Build history of the part. All positions in model axes, mm. A direction names the side the tool comes from. Give positions to 0.01 mm unless a question says otherwise; leave off trailing zeros. Loops run counter-clockwise (first coordinate to the right, second up) from the corner with the lowest first, then second, coordinate; pieces in that order, holes last. Notation, with made-up numbers: (-24.75, 88) -> (31.25, 88) arc R26 ccw to (31.25, 123) -> close; hole circle Ø6 at (-7, 6.5). An arc over 180 degrees is marked (long way). Answer as a JSON object with one key per item and string values. Group by question number.
from build123d import *

# Parameters (mm, degrees)
F0_W     = 98.3068589121
F0_H     = 60.0075013936
F1_DEPTH = 25.4
F2_DEPTH = 25.4
F3_DEPTH = 25.4
F5_DEPTH = 25.4
F7_DEPTH = 58.166


with BuildPart() as f1:
    # F0 (on Front) → F1 (new body)
    with BuildSketch(Plane.XZ):
        with Locations((-25.4295347258, 30.0037506968)):
            Rectangle(F0_W, F0_H)
    extrude(amount=F1_DEPTH)

    # F2 (add): a face of the model
    f2_faces = [f1.faces().sort_by_distance(p)[0] for p in [
        (-25.4295347258, -25.4, 30.0037506968),
    ]]
    extrude(f2_faces, amount=F2_DEPTH)

    # F3 (add): a face of the model
    f3_faces = [f1.faces().sort_by_distance(p)[0] for p in [
        (-74.5829641819, -25.4, 30.0037506968),
    ]]
    extrude(f3_faces, amount=F3_DEPTH)

    # F4 (on face) → F5 (cut)
    with BuildSketch(Plane.XZ.offset(50.8)):
        Polygon((23.7238947302, 60.0075013936), (-69.7281658649, 60.0075013936), (0, 0), (23.7238947302, 0), align=None)
    extrude(amount=-F5_DEPTH, mode=Mode.SUBTRACT)

    # F6 (on face) → F7 (cut)
    with BuildSketch(Plane.XZ.offset(50.8)):
        with BuildLine():
            Line((-18.9269924475, 16.2884181963), (-50.8011734174, 43.7190831973))
            ThreePointArc((-50.8011734174, 43.7190831973), (-48.579415433, 14.0666602118), (-18.9269924475, 16.2884181963))
        make_face()
        with BuildLine():
            ThreePointArc((-18.9269924475, 16.2884181963), (-15.1511722743, 22.6892204926), (-13.8378802624, 30.0037506968))
            ThreePointArc((-13.8378802624, 30.0037506968), (-27.5495527283, 49.716661355), (-50.8011734174, 43.7190831973))
            Line((-50.8011734174, 43.7190831973), (-18.9269924475, 16.2884181963))
        make_face()
    extrude(amount=-F7_DEPTH, mode=Mode.SUBTRACT)


solid = f1.part
(1) 3-axis set-ups, long thin cutter, end or side, ignore diameter. For faces 1 (the flat face through (-51, -14, 60.008)), 2 (the flat face through (-9.6, -38.28, 8.26)): which of +Z, -Z, +X, -X, +Y, -Y reach the whole face in a straight line?
(2) Saw through at A-A on y = -4. List the corners of the cut face in (x, z), plus the area to 3 significant figures.
(3) Probe line 1 along Y through (x, z) = (-2.5, 16); line 2 along X through (y, z) = (-10, 44); line 3 along X through (y, z) = (-24, 12). List the from-to ranges inside material, lowest first. Write a range as [from, to].
(4) Saw through at B-B on x = -40.5. List the corners of the cut face in (y, z).
(5) Pin check, flat tips, straight feed: pin 1 (5 mm diameter, centred on x = -48, y = -32.5, fed in from +Z); pin 2 (1 mm diameter, centred on x = -6, y = -28, fed in from +Z). Stop position of each tip, or through.
(6) Saw through at C-C on z = 35.5. List the corners of the cut face in (x, y).
Calculated:
{
 "1": {"face 1": "+Z, +X, -X, +Y, -Y", "face 2": "+Z, +X, -Y"},
 "2": {"outline": "(-99.98, 0) -> (23.72, 0) -> (23.72, 60.01) -> (-99.98, 60.01) -> close; hole circle Ø42.05 at (-34.86, 30)", "area": "6,030 mm^2"},
 "3": {"line 1": "y = [-25.4, 0]", "line 2": "x = [-99.98, -50.56], [-19.17, 23.72]", "line 3": "x = [-99.98, -45.73], [-24, 23.72]"},
 "4": {"outline": "(-50.8, 0) -> (0, 0) -> (0, 9.75) -> (-50.8, 9.75) -> close; (-25.4, 50.26) -> (0, 50.26) -> (0, 60.01) -> (-25.4, 60.01) -> close"},
 "5": {"pin 1": "stops at z = 15.95", "pin 2": "stops at z = 5.59"},
 "6": {"outline": "(-99.98, -50.8) -> (-55.16, -50.8) -> (-55.16, 0) -> (-99.98, 0) -> close; (-14.57, -25.4) -> (23.72, -25.4) -> (23.72, 0) -> (-14.57, 0) -> close"}
}
